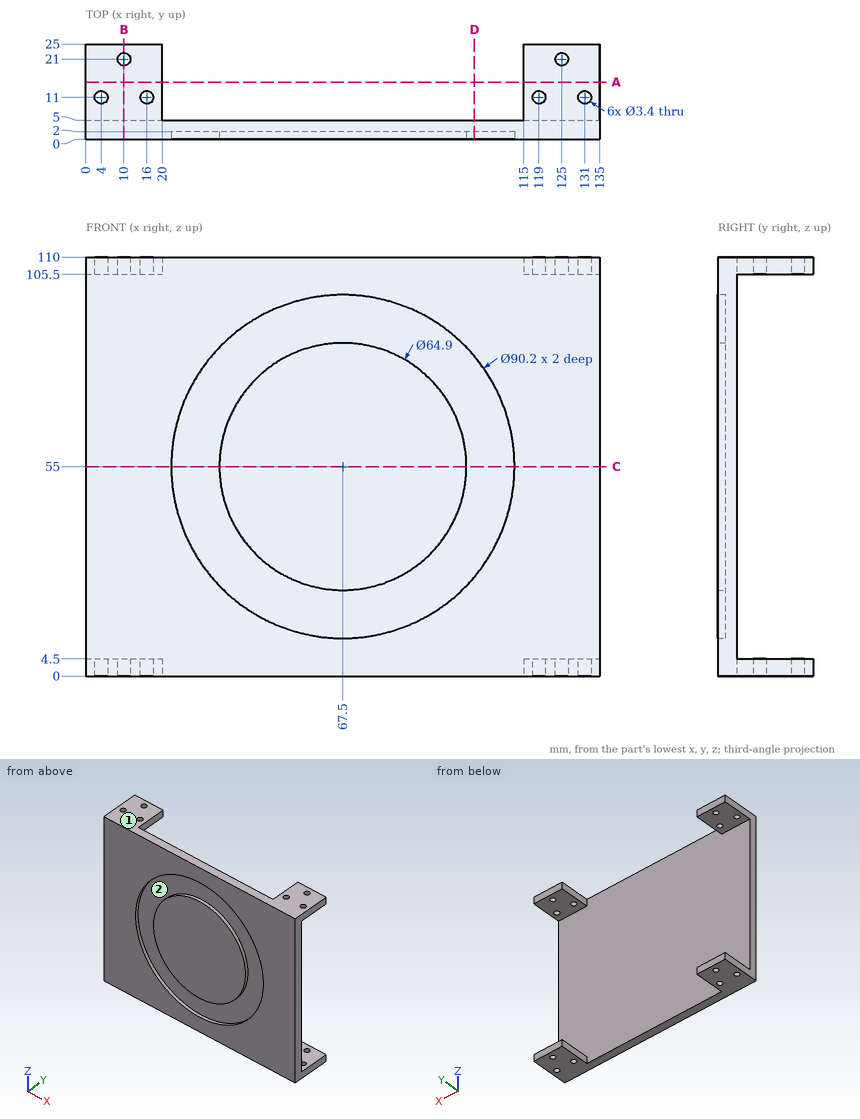
For this review, use the dimensioned drawing (mm, ordinates from the lowest corner) and the shaded views. Round coordinates to 2 decimals unless told otherwise and drop trailing zeros. Write each loop counter-clockwise with the first axis right and the second up, starting at its lowest first coordinate (ties: lowest second). Pieces come first, ordered by that corner, then holes. Notation, with made-up numbers: M 36.5,18 L 43.5,18 A24 ccw 43.5,29 Z; hole C 20.25,16 d1. An arc over 180 degrees is marked long. Use CSV: the item, a comma, the result in double quotes. Start each with the question number.
(1) We need section D-D, the plane x = 102. State the section outline as (y, z) points, then the cut area to 3 significant figures.
(2) We need section B-B, the plane x = 10. State the section outline as (y, z) points.
(3) For line 1 along Z through (x, y) = (116, 9.75); line 2 along Y through (x, z) = (16, 3.45); line 3 along Y through (x, z) = (125, 6), list the stretches that pass through material, from the lowest coordinate up.
(4) The part is to be moulded in two halves that separate along X. For the marked faces 1 and 2, say which applies: +X half, -X half, draft (parallel to the pull), parting line (faces both ways), or undercut.
(5) Clearance check with flat-ended pins moving along their axes: P1, Ø2, axis at x = 16, y = 11, coming from the +Z side; P2, Ø12, axis at x = 24, y = 9, coming from the -Z side; P3, Ø5, axis at x = 70, z = 87, coming from the +Y side. State where each tip first meets the part, or that it passes through.
(6) We need section C-C, the plane z = 55. State the section outline as (x, y) points.
(7) We need section A-A, the plane y = 15. State the section outline as (x, z) points.
Findings:
1,outline,"M 0,0 L 5,0 L 5,110 L 0,110 L 0,84.05 L 2,84.05 L 2,25.95 L 0,25.95 Z"
1,area,"434 mm^2"
2,outline,"M 0,0 L 19.3,0 L 19.3,4.5 L 5,4.5 L 5,105.5 L 19.3,105.5 L 19.3,110 L 0,110 Z; M 22.7,0 L 25,0 L 25,4.5 L 22.7,4.5 Z; M 22.7,105.5 L 25,105.5 L 25,110 L 22.7,110 Z"
3,line 1,"0 to 4.5, 105.5 to 110"
3,line 2,"0 to 9.3, 12.7 to 25"
3,line 3,"0 to 5"
4,face 1,"draft"
4,face 2,"undercut"
5,P1,"through"
5,P2,"z = 0"
5,P3,"y = 5"
6,outline,"M 0,0 L 22.4,0 L 22.4,2 L 35.05,2 L 35.05,0 L 99.95,0 L 99.95,2 L 112.6,2 L 112.6,0 L 135,0 L 135,5 L 0,5 Z"
7,outline,"M 0,0 L 20,0 L 20,4.5 L 0,4.5 Z; M 0,105.5 L 20,105.5 L 20,110 L 0,110 Z; M 115,0 L 135,0 L 135,4.5 L 115,4.5 Z; M 115,105.5 L 135,105.5 L 135,110 L 115,110 Z"
